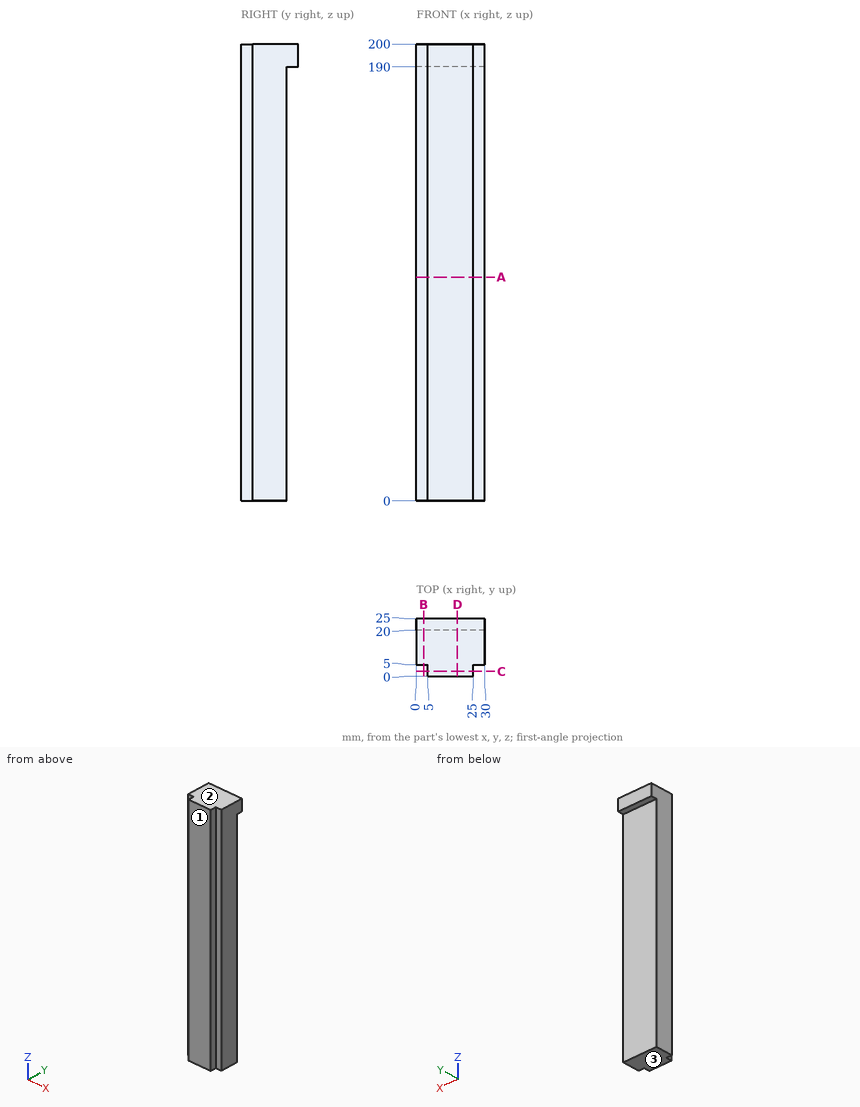
Drawing for the job (mm, zero at the part's lowest x, y, z). Give positions to 0.01 mm unless a question says otherwise; leave off trailing zeros. Write each loop counter-clockwise with the first axis right and the second up, starting at its lowest first coordinate (ties: lowest second). Pieces come first, ordered by that corner, then holes. Notation, with made-up numbers: (40, 17) -> (68, 17) arc R22 ccw to (68, 41) -> close; hole circle Ø2 at (-35.5, -9). An arc over 180 degrees is marked (long way). Put each result on its own line as item: value. Start each with the question number.
Item 1: Wall check: L1, parallel to Y at x = 26.5, z = 11.5; L2, parallel to Y at x = 15.5, z = 56; L3, parallel to Z at x = 5.25, y = 23.5. Give the ranges that are in metal, low to high. Write a range as [from, to].
Item 2: Pin check, flat tips, straight feed: pin 1 Ø1.5 at (x, z) = (2, 111.5) entering from -Y; pin 2 Ø4 at (x, y) = (11, 17) entering from -Z; pin 3 Ø1.5 at (y, z) = (2, 141) entering from -X; pin 4 Ø5.5 at (y, z) = (2, 120) entering from +X. Stop position of each tip, or through.
Item 3: Pull direction Z, two halves, no side cores. Call the marked faces 1, 2 and 3: pulls with the +Z half, pulls with the -Z half, needs draft (parallel to the pull), parting line crosses it, or undercut.
Item 4: Cut at A-A (z = 98). List the corners of the cut face in (x, y), then the cut area to 3 significant figures.
Item 5: Cut at D-D (x = 18). List the corners of the cut face in (y, z).
Item 6: Cut at B-B (x = 3.25). List the corners of the cut face in (y, z).
Item 7: Cut at C-C (y = 2). List the corners of the cut face in (x, z), then the cut area to 3 significant figures.
Answer list:
1. L1: y = [5, 20]
1. L2: y = [0, 20]
1. L3: z = [190, 200]
2. pin 1: stops at y = 5
2. pin 2: stops at z = 0
2. pin 3: stops at x = 5
2. pin 4: stops at x = 25
3. face 1: needs draft
3. face 2: pulls with the +Z half
3. face 3: pulls with the -Z half
4. outline: (0, 5) -> (5, 5) -> (5, 0) -> (25, 0) -> (25, 5) -> (30, 5) -> (30, 20) -> (0, 20) -> close
4. area: 550 mm2
5. outline: (0, 0) -> (20, 0) -> (20, 190) -> (25, 190) -> (25, 200) -> (0, 200) -> close
6. outline: (5, 0) -> (20, 0) -> (20, 190) -> (25, 190) -> (25, 200) -> (5, 200) -> close
7. outline: (5, 0) -> (25, 0) -> (25, 200) -> (5, 200) -> close
7. area: 4,000 mm2
